```python
from build123d import *

# Parameters (mm, degrees)
F0_W     = 263
F0_H     = 308
F1_DEPTH = 108.5
F2_R     = 34.2595
F3_DEPTH = 25
F4_T     = -2.5
F5_R     = 5


with BuildPart() as f1:
    # F0 (on Top) → F1 (new body)
    with BuildSketch(Plane.XY):
        Rectangle(F0_W, F0_H)
    extrude(amount=F1_DEPTH)

    # F2 (on face) → F3 (join)
    with BuildSketch(Plane.YZ.offset(131.5)):
        with Locations((76.1949643493, 52.8052560985)):
            Circle(F2_R)
    extrude(amount=F3_DEPTH)

    # F4
    f4_openings = [f1.faces().sort_by_distance(p)[0] for p in [
        (156.5, 76.194964, 52.805256),
    ]]
    offset(amount=F4_T, openings=f4_openings, kind=Kind.INTERSECTION)

    # F5
    f5_edges = [f1.edges().sort_by_distance(p)[0] for p in [
        (0, 154, 108.5),
        (0, -154, 108.5),
        (0, 154, 0),
        (0, -154, 0),
        (131.5, 0, 108.5),
        (131.5, 0, 0),
        (-131.5, 0, 108.5),
        (-131.5, 0, 0),
    ]]
    fillet(f5_edges, radius=F5_R)


solid = f1.part
```
Verification items for the finished model (mm, model axes). A direction names the side the tool comes from. Coordinates: 2 decimals unless noted, no trailing zeros. Loops run counter-clockwise (first coordinate to the right, second up) from the corner with the lowest first, then second, coordinate; pieces in that order, holes last. Notation, with made-up numbers: (-9, -28) - (47, -28) arc R15 cw to (47, -17) - close; hole circle Ø6 at (11.25, 68.5). An arc over 180 degrees is marked (long way). Answer as a JSON object with one key per item and string values.
(1) Mould release check, pull along Y, two halves, no side actions. Record for faces 1 (the flat face through (-2, 154, 54)), 2 (the flat face through (-2, 2, 0)), 3 (the flat face through (-2, 2, 2.5)): pulls with the +Y half, pulls with the -Y half, needs draft (parallel to the pull), parting line crosses it, or undercut.
Response:
{"face 1": "pulls with the +Y half", "face 2": "needs draft", "face 3": "undercut"}
(2) Cross-section at C-C, the plane x = 24. Record the boundary of the cut face in (y, z), then the cut area to 3 significant figures.
Response:
{"outline": "(-154, 5) arc R5 ccw to (-149, 0) - (149, 0) arc R5 ccw to (154, 5) - (154, 103.5) arc R5 ccw to (149, 108.5) - (-149, 108.5) arc R5 ccw to (-154, 103.5) - close; hole (-151.5, 2.5) - (151.5, 2.5) - (151.5, 106) - (-151.5, 106) - close", "area": "2,040 mm²"}
(3) Cross-section at A-A, the plane z = 97.5. Record the boundary of the cut face in (x, y), then the cut area to 3 significant figures.
Response:
{"outline": "(-131.5, -154) - (131.5, -154) - (131.5, 154) - (-131.5, 154) - close; hole (-129, -151.5) - (129, -151.5) - (129, 151.5) - (-129, 151.5) - close", "area": "2,830 mm²"}
(4) Go/stop test with a flat-tipped pin: pin 1 Ø10 at (y, z) = (36.5, 16.5) entering from +X. Record where the tip stops, or that it passes through.
Response:
{"pin 1": "stops at x = 131.5"}
(5) Cross-section at B-B, the plane y = -82.5. Record the boundary of the cut face in (x, z), then the cut area to 3 significant figures.
Response:
{"outline": "(-131.5, 5) arc R5 ccw to (-126.5, 0) - (126.5, 0) arc R5 ccw to (131.5, 5) - (131.5, 103.5) arc R5 ccw to (126.5, 108.5) - (-126.5, 108.5) arc R5 ccw to (-131.5, 103.5) - close; hole (-129, 2.5) - (129, 2.5) - (129, 106) - (-129, 106) - close", "area": "1,810 mm²"}
(6) Access from +Z, -Z, +X, -X, +Y, -Y to the whole of each face (thin tool, end or side, straight path). Record for faces 4 (the flat face through (-2, 2, 108.5)), 5 (the cylindrical face through (143.825, 49.008, 31.959)), 6 (the flat face through (-2, -151.5, 54)).
Response:
{"face 4": "+Z, +X, -X, +Y, -Y", "face 5": "+X", "face 6": "none"}
(7) Scan lines: line 1 along Z through (x, y) = (-88, -9); line 2 along Y through (x, z) = (118.5, 87); line 3 along X through (y, z) = (-10, 79). Record each from-to range of solid material in increasing order.
Response:
{"line 1": "z = 0 to 2.5, 106 to 108.5", "line 2": "y = -154 to -151.5, 151.5 to 154", "line 3": "x = -131.5 to -129, 129 to 131.5"}
(8) Cross-section at D-D, the plane y = 91. Record the boundary of the cut face in (x, z), then the cut area to 3 significant figures.
Response:
{"outline": "(-131.5, 5) arc R5 ccw to (-126.5, 0) - (126.5, 0) arc R5 ccw to (131.5, 5) - (131.5, 21.91) - (156.5, 21.91) - (156.5, 24.71) - (129, 24.71) - (129, 2.5) - (-129, 2.5) - (-129, 106) - (129, 106) - (129, 80.9) - (156.5, 80.9) - (156.5, 83.7) - (131.5, 83.7) - (131.5, 103.5) arc R5 ccw to (126.5, 108.5) - (-126.5, 108.5) arc R5 ccw to (-131.5, 103.5) - close", "area": "1,810 mm²"}
